The listing builds one solid part. Answer for the finished solid, in the listing's coordinates (mm). A direction names the side the tool comes from. Coordinates: 2 decimals unless noted, no trailing zeros. Write each loop counter-clockwise with the first axis right and the second up, starting at its lowest first coordinate (ties: lowest second). Pieces come first, ordered by that corner, then holes.
(1) Which of the six approach directions +Z, -Z, +X, -X, +Y, -Y give full straight-line access (tool end or side, diameter ignored) to faces 1 (the flat face through (-115.161, -1, 25)), 2 (the flat face through (-12, -55, 25)), 3 (the cylindrical face through (45.108, 55.223, 48.521))?
(2) The part is cut by section B-B on z = 28. Determine the outline of the cut face in (x, y), plus the area to 3 significant figures.
(3) The part is cut by section A-A on x = -17.5. Determine the outline of the cut face in (y, z).
(4) Given P1, Ø3, axis at x = -87.66, y = -47.5, coming from the -Z side, flat-ended and moving along its own axis, determine where the tip first touches the part or whether it passes through.
(5) The part is cut by section D-D on y = -7. Determine the outline of the cut face in (x, z), plus the area to 3 significant figures.
(6) Straight lines are drawn through the part: line 1 (X direction, y = -47.5, z = 1.1); line 2 (Z direction, x = -17, y = 3); line 3 (Y direction, x = -27, z = 31). For each, find the intervals that lie inside material, in ascending order.
(7) The part is cut by section C-C on y = 23. Determine the outline of the cut face in (x, z), plus the area to 3 significant figures.
(8) For a pull along X with two mould halves and no side action, classify faces 4 (the flat face through (-12, 1, 0)), 5 (the flat face through (-12, 1, 2.5)), 6 (the flat face through (-112.661, -1, 25)), 7 (the flat face through (94.839, -1, 25)) as +X half, -X half, draft (parallel to the pull), parting line (faces both ways), or undercut.
from build123d import *

# Parameters (mm, degrees)
F0_W     = 210
F0_H     = 115
F1_DEPTH = 50
F3_T     = -2.5
F2_R     = 32.5
F4_DEPTH = 3
F6_D     = 3.4
F6_DEPTH = 4
F6_TIP   = 1.0214630523


with BuildPart() as f1:
    # F0 (on Top) → F1 (new body)
    with BuildSketch(Plane.XY):
        with Locations((-10.1612838779, 0)):
            Rectangle(F0_W, F0_H)
    extrude(amount=F1_DEPTH)

    # F3 (hollow: no face is removed)
    offset(amount=F3_T, mode=Mode.SUBTRACT)

    # F2 (on face) → F4 (cut)
    with BuildSketch(Plane.XY.offset(50)):
        with Locations((49.3387161221, 23)):
            Circle(F2_R)
    extrude(amount=-F4_DEPTH, mode=Mode.SUBTRACT)

    # F6
    with Locations(Plane(origin=(0, 0, 0), x_dir=(1, 0, 0), z_dir=(0, 0, -1))):
        with Locations((-87.6612838779, 47.5), (89.8387161221, 47.5), (89.8387161221, -47.5), (-87.6612838779, -47.5)):
            Hole(F6_D / 2, depth=F6_DEPTH)
            with Locations((0, 0, -(F6_DEPTH + F6_TIP / 2))):  # 118° drill point
                Cone(0, F6_D / 2, F6_TIP, mode=Mode.SUBTRACT)


solid = f1.part
Model answer:
1. face 1: +Z, -Z, -X, +Y, -Y
1. face 2: none
1. face 3: +Z
2. outline: (-115.16, -57.5) - (94.84, -57.5) - (94.84, 57.5) - (-115.16, 57.5) - close; hole (-112.66, -55) - (92.34, -55) - (92.34, 55) - (-112.66, 55) - close
2. area: 1,600 mm2
3. outline: (-57.5, 0) - (57.5, 0) - (57.5, 50) - (-57.5, 50) - close; hole (-55, 2.5) - (55, 2.5) - (55, 47.5) - (-55, 47.5) - close
4. P1: stops at z = 47.5
5. outline: (-115.16, 0) - (94.84, 0) - (94.84, 50) - (61.84, 50) - (61.84, 47.5) - (92.34, 47.5) - (92.34, 2.5) - (-112.66, 2.5) - (-112.66, 47.5) - (36.84, 47.5) - (36.84, 50) - (-115.16, 50) - close
5. area: 1,210 mm2
6. line 1: x = -115.16 to -89.36, -85.96 to 88.14, 91.54 to 94.84
6. line 2: z = 0 to 2.5, 47.5 to 50
6. line 3: y = -57.5 to -55, 55 to 57.5
7. outline: (-115.16, 0) - (94.84, 0) - (94.84, 50) - (81.84, 50) - (81.84, 47.5) - (92.34, 47.5) - (92.34, 2.5) - (-112.66, 2.5) - (-112.66, 47.5) - (16.84, 47.5) - (16.84, 50) - (-115.16, 50) - close
7. area: 1,110 mm2
8. face 4: draft
8. face 5: undercut
8. face 6: undercut
8. face 7: +X half
